Geometry: final body of the model. Coordinates: model frame, mm. Face numbers are marked on the shaded views. A direction names the side the tool comes from. Round coordinates to 2 decimals unless told otherwise and drop trailing zeros. Loops run counter-clockwise (first coordinate to the right, second up) from the corner with the lowest first, then second, coordinate; pieces in that order, holes last. Notation, with made-up numbers: (-18.75, -7.5) - (39.25, -7.5) arc R17 cw to (39.25, 0.5) - close; hole circle Ø9 at (17.25, 18.25). An arc over 180 degrees is marked (long way). Answer as CSV lines item,"result".
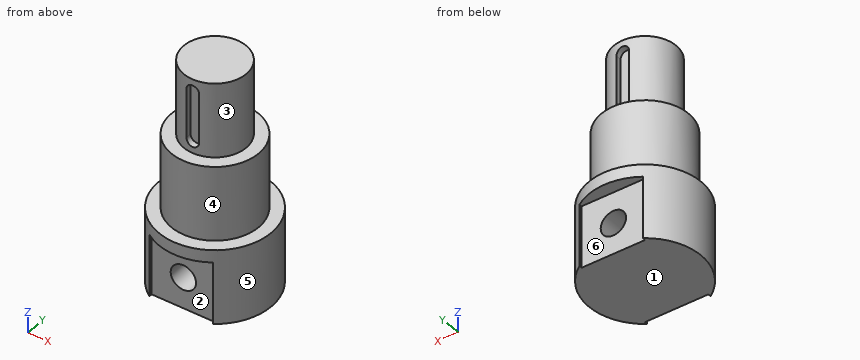
from build123d import *

# Parameters (mm, degrees)
CROQUIS1_R              = 18
SALIENTE_EXTRUIR1_DEPTH = 24
CROQUIS2_R              = 14
SALIENTE_EXTRUIR2_DEPTH = 24
CROQUIS3_R              = 10
SALIENTE_EXTRUIR3_DEPTH = 24
CORTAR_EXTRUIR1_DEPTH   = 2
CORTAR_EXTRUIR2_DEPTH   = 2
CROQUIS6_W              = 20
CROQUIS6_H              = 20
CORTAR_EXTRUIR3_DEPTH   = 4
CROQUIS7_W              = 20
CROQUIS7_H              = 20
CORTAR_EXTRUIR4_DEPTH   = 4
CROQUIS8_R              = 4
CORTAR_EXTRUIR5_DEPTH   = 33


with BuildPart() as part:
    # Croquis1 → Saliente-Extruir1 (new body)
    with BuildSketch(Plane.XY):
        Circle(CROQUIS1_R)
    extrude(amount=SALIENTE_EXTRUIR1_DEPTH)

    # Croquis2 → Saliente-Extruir2 (add)
    with BuildSketch(Plane.XY.offset(24)):
        Circle(CROQUIS2_R)
    extrude(amount=SALIENTE_EXTRUIR2_DEPTH)

    # Croquis3 → Saliente-Extruir3 (add)
    with BuildSketch(Plane.XY.offset(48)):
        Circle(CROQUIS3_R)
    extrude(amount=SALIENTE_EXTRUIR3_DEPTH)

    # Croquis4 → Cortar-Extruir1 (cut)
    with BuildSketch(Plane(origin=(0, 10, 0), x_dir=(1, 0, 0), z_dir=(0, 1, 0))):
        with BuildLine():
            Line((2, -52), (2, -68))
            ThreePointArc((2, -68), (0, -70), (-2, -68))
            Line((-2, -68), (-2, -52))
            ThreePointArc((-2, -52), (0, -50), (2, -52))
        make_face()
    extrude(amount=-CORTAR_EXTRUIR1_DEPTH, mode=Mode.SUBTRACT)

    # Croquis5 → Cortar-Extruir2 (cut)
    with BuildSketch(Plane(origin=(0, -10, 0), x_dir=(1, 0, 0), z_dir=(0, 1, 0))):
        with BuildLine():
            Line((-2, -68), (-2, -52))
            ThreePointArc((-2, -52), (0, -50), (2, -52))
            Line((2, -52), (2, -68))
            ThreePointArc((2, -68), (0, -70), (-2, -68))
        make_face()
    extrude(amount=CORTAR_EXTRUIR2_DEPTH, mode=Mode.SUBTRACT)

    # Croquis6 → Cortar-Extruir3 (cut)
    with BuildSketch(Plane(origin=(0, 18, 0), x_dir=(1, 0, 0), z_dir=(0, 1, 0))):
        with Locations((0, -10)):
            Rectangle(CROQUIS6_W, CROQUIS6_H)
    extrude(amount=-CORTAR_EXTRUIR3_DEPTH, mode=Mode.SUBTRACT)

    # Croquis7 → Cortar-Extruir4 (cut)
    with BuildSketch(Plane(origin=(0, -18, 0), x_dir=(1, 0, 0), z_dir=(0, 1, 0))):
        with Locations((0, -10)):
            Rectangle(CROQUIS7_W, CROQUIS7_H)
    extrude(amount=CORTAR_EXTRUIR4_DEPTH, mode=Mode.SUBTRACT)

    # Croquis8 → Cortar-Extruir5 (cut, through all)
    with BuildSketch(Plane.XZ.offset(14)):
        with Locations((0, 10)):
            Circle(CROQUIS8_R)
    extrude(amount=-CORTAR_EXTRUIR5_DEPTH, mode=Mode.SUBTRACT)


solid = part.part
(1) Draft query along X for the marked faces 1, 2 and 3. Return one class per face: pulls with the +X half, pulls with the -X half, needs draft (parallel to the pull), parting line crosses it, or undercut.
Findings below:
face 1,"needs draft"
face 2,"undercut"
face 3,"parting line crosses it"
(2) Access query for the marked faces 4, 5 and 6. Directions: +Z, -Z, +X, -X, +Y, -Y. A direction counts if a zero-diameter tool reaches every point of the face in a straight line with its end or side. Return the directions, or none.
Findings below:
face 4,"+Z"
face 5,"+Z, -Z"
face 6,"-Z, +Y"
(3) Section B-B (x = 0). Output: boundary loops of the cut face in (y, z).
Findings below:
outline,"(-18, 20) - (-14, 20) - (-14, 14) - (14, 14) - (14, 20) - (18, 20) - (18, 24) - (14, 24) - (14, 48) - (10, 48) - (10, 50) - (8, 50) - (8, 70) - (10, 70) - (10, 72) - (-10, 72) - (-10, 70) - (-8, 70) - (-8, 50) - (-10, 50) - (-10, 48) - (-14, 48) - (-14, 24) - (-18, 24) - close; (-14, 0) - (14, 0) - (14, 6) - (-14, 6) - close"
(4) Section D-D (x = -9). Output: boundary loops of the cut face in (y, z), and give its area (3 significant figures).
Findings below:
outline,"(-15.59, 20) - (-14, 20) - (-14, 0) - (14, 0) - (14, 20) - (15.59, 20) - (15.59, 24) - (10.72, 24) - (10.72, 48) - (4.36, 48) - (4.36, 72) - (-4.36, 72) - (-4.36, 48) - (-10.72, 48) - (-10.72, 24) - (-15.59, 24) - close"
area,"1,410 mm2"
(5) Section A-A (z = 10). Output: boundary loops of the cut face in (x, y), and give its area (3 significant figures).
Findings below:
outline,"(-10, -14.97) - (-10, -14) - (-4, -14) - (-4, 14) - (-10, 14) - (-10, 14.97) arc R18 ccw to start; (4, -14) - (10, -14) - (10, -14.97) arc R18 ccw to (10, 14.97) - (10, 14) - (4, 14) - close"
area,"673 mm2"
(6) Material intervals for line 1 along Z through (x, y) = (0, 7.25); line 2 along Z through (x, y) = (8.5, -8.5); line 3 along Y through (x, z) = (1, 55.5), sorted ascending.
Findings below:
line 1,"0 to 6, 14 to 72"
line 2,"0 to 48"
line 3,"-8 to 8"
(7) Pin query (flat end, axial travel): P1, Ø12, axis at x = -14, y = 2, coming from the -Z side; P2, Ø6, axis at x = 2.5, z = 7, coming from the +Y side; P3, Ø1.4, axis at y = -8.5, z = 64, coming from the -X side; P4, Ø4.5, axis at x = -1, z = 63.5, coming from the -Y side. Return the tip coordinate at first contact, or that it passes through.
Findings below:
P1,"z = 0"
P2,"y = 14"
P3,"x = -6.26"
P4,"y = -9.8"
(8) Section C-C (y = 0). Output: boundary loops of the cut face in (x, z), and give its area (3 significant figures).
Findings below:
outline,"(-18, 0) - (18, 0) - (18, 24) - (14, 24) - (14, 48) - (10, 48) - (10, 72) - (-10, 72) - (-10, 48) - (-14, 48) - (-14, 24) - (-18, 24) - close; hole circle Ø8 at (0, 10)"
area,"1,970 mm2"
